from build123d import *

# Parameters (mm, degrees)
SALIENTE_EXTRUIR1_DEPTH = 2.5
SALIENTE_EXTRUIR2_START = 7
SALIENTE_EXTRUIR2_DEPTH = 7
SALIENTE_EXTRUIR3_START = 7.5
CROQUIS2_4_R            = 10
SALIENTE_EXTRUIR3_DEPTH = 7.5
REDONDEO1_R             = 4
REDONDEO2_R             = 4
CROQUIS3_R              = 10
SALIENTE_EXTRUIR4_DEPTH = 5
CROQUIS4_R              = 5.05
CORTAR_EXTRUIR1_DEPTH   = 131
CROQUIS5_R              = 5.78
CORTAR_EXTRUIR2_DEPTH   = 1.5


with BuildPart() as part:
    # Croquis2 → Saliente-Extruir1 (new, symmetric)
    with BuildSketch(Plane(origin=(0, 0, 0), x_dir=(0, 0, -1), z_dir=(1, 0, 0))):
        with BuildLine():
            ThreePointArc((31.95, 0), (22.592061659, 22.592061659), (0, 31.95))
            Line((0, 31.95), (0, 0))
            Line((0, 0), (31.95, 0))
        make_face()
    extrude(amount=SALIENTE_EXTRUIR1_DEPTH, both=True)

    # Croquis2<3> → Saliente-Extruir2 (add)
    with BuildSketch(Plane(origin=(0, 0, 0), x_dir=(0, 0, -1), z_dir=(1, 0, 0)).offset(SALIENTE_EXTRUIR2_START)):
        with BuildLine():
            ThreePointArc((10, 53.9), (7.071067812, 46.828932188), (0, 43.9))
            Line((0, 43.9), (0, 31.95))
            ThreePointArc((0, 31.95), (22.592061659, 22.592061659), (31.95, 0))
            Line((31.95, 0), (43.9, 0))
            ThreePointArc((43.9, 0), (53.9, 10), (63.9, 0))
            ThreePointArc((63.9, 0), (45.184123318, 45.184123318), (0, 63.9))
            ThreePointArc((0, 63.9), (7.071067812, 60.971067812), (10, 53.9))
        make_face()
    extrude(amount=-SALIENTE_EXTRUIR2_DEPTH)

    # Croquis2<4> → Saliente-Extruir3 (add)
    with BuildSketch(Plane(origin=(0, 0, 0), x_dir=(0, 0, -1), z_dir=(1, 0, 0)).offset(SALIENTE_EXTRUIR3_START)):
        with Locations(Location((0, 53.9, 0), (0, 0, 270))):
            Circle(CROQUIS2_4_R)
        with Locations((53.9, 0)):
            Circle(CROQUIS2_4_R)
    extrude(amount=-SALIENTE_EXTRUIR3_DEPTH)

    # Redondeo1
    redondeo1_edges = [part.edges().sort_by_distance(p)[0] for p in [
        (0, 0, 0),
    ]]
    fillet(redondeo1_edges, radius=REDONDEO1_R)

    # Redondeo2
    # the kernel refuses this fillet: 4 mm, written as the material it adds along each edge
    with BuildSketch(Plane(origin=(7, 0, -43.9), x_dir=(0, 0, 1), z_dir=(-1, 0, 0))) as redondeo2_piece_1:
        with BuildLine():
            CenterArc((3.416407865, -4), REDONDEO2_R, 90, 73.398450401)
            ThreePointArc((-0.416851525, -2.857142857), (-0.104761631, -1.443695821), (0, 0))
            Line((0, 0), (3.416407865, 0))
        make_face()
    extrude(amount=7)
    with BuildSketch(Plane(origin=(7, 43.9, 0), x_dir=(0, -1, 0), z_dir=(-1, 0, 0))) as redondeo2_piece_2:
        with BuildLine():
            CenterArc((3.416407865, 4), REDONDEO2_R, 196.601549599, 73.398450401)
            ThreePointArc((-0.416851525, 2.857142857), (-0.104761631, 1.443695821), (0, 0))
            Line((0, 0), (3.416407865, 0))
        make_face()
    extrude(amount=7)

    # Croquis3 → Saliente-Extruir4 (add)
    with BuildSketch(Plane(origin=(2.5, 0, 0), x_dir=(0, 0, -1), z_dir=(1, 0, 0))):
        with Locations((4, 4)):
            Circle(CROQUIS3_R)
    extrude(amount=-SALIENTE_EXTRUIR4_DEPTH)

    # Croquis4 → Cortar-Extruir1 (cut)
    with BuildSketch(Plane(origin=(2.5, 0, 0), x_dir=(0, 0, -1), z_dir=(1, 0, 0))):
        with Locations((4, 4)):
            Circle(CROQUIS4_R)
    extrude(amount=-CORTAR_EXTRUIR1_DEPTH, mode=Mode.SUBTRACT)

    # Croquis5 → Cortar-Extruir2 (cut)
    with BuildSketch(Plane.ZY.offset(2.5)):
        with Locations((-4, 4)):
            Circle(CROQUIS5_R)
    extrude(amount=-CORTAR_EXTRUIR2_DEPTH, mode=Mode.SUBTRACT)


solid = part.part
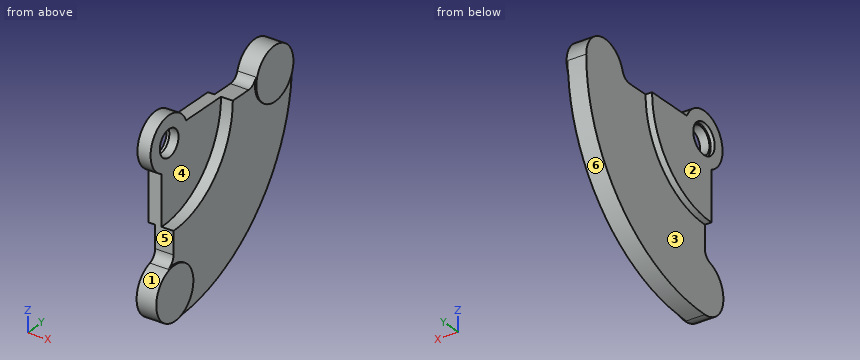
Geometry check sheet. Reference: the model listing, model coordinates, mm. Face numbers are marked on the shaded views. A direction names the side the tool comes from. Give positions to 0.01 mm unless a question says otherwise; leave off trailing zeros. Order: outer loops, then holes, each group sorted by start corner. A loop starts at its lowest first (then second) coordinate and runs counter-clockwise, first axis right, second up. Notation, with made-up numbers: M -21.75,-28 L 3.25,-28 A31 ccw 3.25,11 Z; hole C -16.5,45.5 d4. An arc over 180 degrees is marked long. Use a Markdown table: item, result.
Item 1: Tool access check on the marked faces 1, 2 and 3. Record the directions out of +Z, -Z, +X, -X, +Y, -Y that give a thin tool (end or side, any length) a straight path to the whole face; none if there is none.
Answers follow:
| item | result |
|---|---|
| face 1 | +X |
| face 2 | +Z, -Z, -X, +Y, -Y |
| face 3 | -Z, -X, +Y |
Item 2: Material ranges on line 1 along X through (y, z) = (10.5, -34); line 2 along Y through (x, z) = (-0.25, -4); line 3 along Y through (x, z) = (-2.05, -4), recorded low to high.
Answers follow:
| item | result |
|---|---|
| line 1 | x = 0 to 7 |
| line 2 | y = -6 to -1.05, 9.05 to 31.7 |
| line 3 | y = -6 to -1.78, 9.78 to 31.7 |
Item 3: Section check C-C (y = 4). Record the cut outline in (x, z).
Answers follow:
| item | result |
|---|---|
| outline | M -2.5,-31.7 L 0,-31.7 L 0,-63.77 L 7,-63.77 L 7,-63.07 L 7.5,-63.07 L 7.5,-44.73 L 7,-44.73 L 7,-31.7 L 2.5,-31.7 L 2.5,-9.05 L -1,-9.05 L -1,-9.78 L -2.5,-9.78 Z; M -2.5,1.78 L -1,1.78 L -1,1.05 L 2.5,1.05 L 2.5,6 L -2.5,6 Z |
Item 4: Section check A-A (z = -4). Record the cut outline in (x, y), and give its area (4 significant figures).
Answers follow:
| item | result |
|---|---|
| outline | M -2.5,-6 L 2.5,-6 L 2.5,-1.05 L -1,-1.05 L -1,-1.78 L -2.5,-1.78 Z; M -2.5,9.78 L -1,9.78 L -1,9.05 L 2.5,9.05 L 2.5,31.7 L 7,31.7 L 7,44.73 L 7.5,44.73 L 7.5,63.07 L 7,63.07 L 7,63.77 L 0,63.77 L 0,31.7 L -2.5,31.7 Z |
| area | 369.5 mm2 |
Item 5: Section check D-D (z = -23.5). Record the cut outline in (x, y).
Answers follow:
| item | result |
|---|---|
| outline | M -2.5,0 L 2.5,0 L 2.5,21.65 L 7,21.65 L 7,59.42 L 0,59.42 L 0,21.65 L -2.5,21.65 Z |
Item 6: Draft check along Z on the marked faces 4, 5 and 6. Enter one of: +Z half, -Z half, draft (parallel to the pull), parting line (faces both ways), or undercut.
Answers follow:
| item | result |
|---|---|
| face 4 | draft |
| face 5 | undercut |
| face 6 | -Z half |
Item 7: Depth check by flat-ended pin: P1, Ø5, axis at y = 40.5, z = -23, coming from the +X side; P2, Ø1, axis at x = 5.5, y = 52, coming from the -Z side; P3, Ø5, axis at x = 1.5, y = 25, coming from the +Z side. Enter the tip coordinate at first touch or a pass-through.
Answers follow:
| item | result |
|---|---|
| P1 | stops at x = 7 |
| P2 | stops at z = -37.83 |
| P3 | stops at z = 0 |
Item 8: Section check B-B (y = 15.5). Record the cut outline in (x, z).
Answers follow:
| item | result |
|---|---|
| outline | M -2.5,-27.94 L 0,-27.94 L 0,-61.99 L 7,-61.99 L 7,-27.94 L 2.5,-27.94 L 2.5,0 L -2.5,0 Z |
